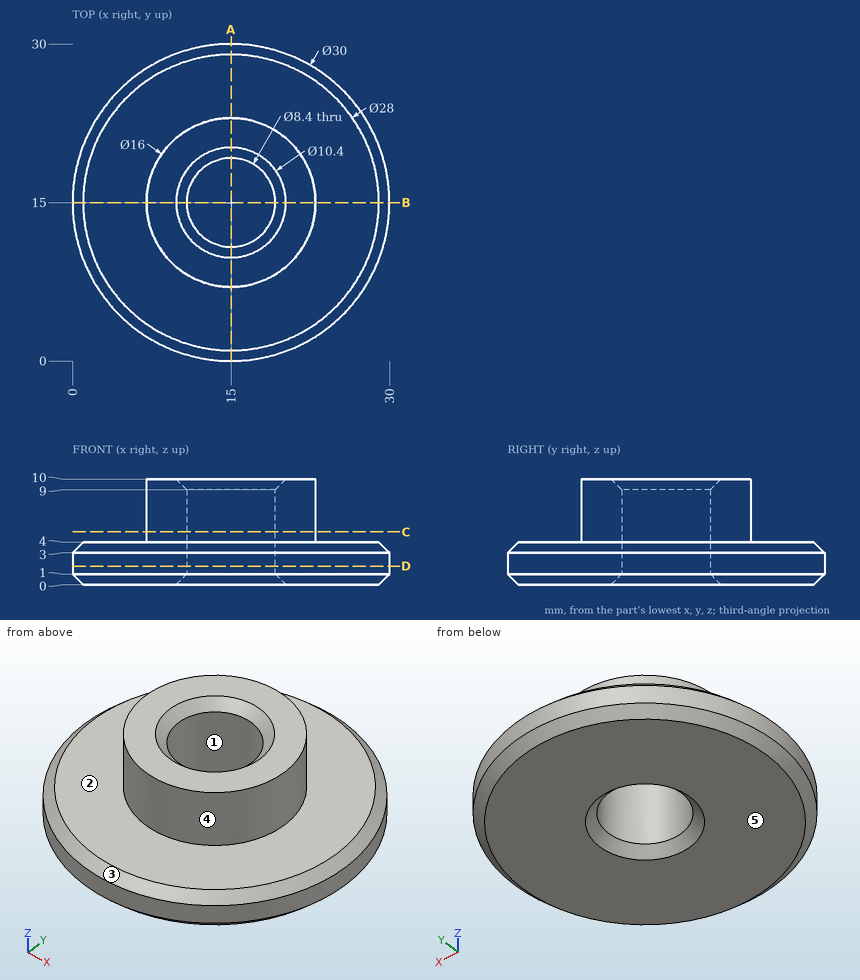
Study the drawing (mm; zero at the part's minimum x, y, z) and answer. A direction names the side the tool comes from. Give positions to 0.01 mm unless a question says otherwise; leave off trailing zeros. Loops run counter-clockwise (first coordinate to the right, second up) from the corner with the lowest first, then second, coordinate; pieces in that order, holes last. Notation, with made-up numbers: (80.5, 49.25) - (86.5, 49.25) arc R18 cw to (86.5, 53.25) - close; hole circle Ø8 at (33.25, 0.5). An arc over 180 degrees is marked (long way). Answer in a Markdown table with one row per item. Add a question column.
Q1. The part is cut by section C-C (z = 5). Determine the outline of the cut face in (x, y).
Q2. The part is cut by section D-D (z = 1.75). Determine the outline of the cut face in (x, y), and give its area (3 significant figures).
Q3. Determine the mould class of the marked faces 1, 2 and 3 for opening direction X: released by +X, released by -X, zero draft, split by the parting line, or undercut.
Q4. The part is cut by section A-A (x = 15). Determine the outline of the cut face in (y, z).
Q5. Consider line 1 along Y through (x, z) = (15, 4.75); line 2 along Z through (x, y) = (19.25, 23); line 3 along Y through (x, z) = (16.5, 5.5). Determine where each line is inside the solid, lowest interval first.
Q6. Each of these flat-tipped pins is pushed along its axis until it touches: P1, Ø6, axis at x = 3.5, y = 15.5, coming from the +Z side; P2, Ø6, axis at x = 18.5, z = 3, coming from the +Y side; P3, Ø1.5, axis at x = 12, z = 2.5, coming from the +Y side. Where does it stop, or does it pass through?
Q7. A tool of negligible diameter and unlimited length cuts with its end or side. For the marked faces 4 and 5, from which of +Z, -Z, +X, -X, +Y, -Y can it reach the whole face along a straight path? Write none if from no direction.
Solution:
| question | item | result |
|---|---|---|
| 1 | outline | circle Ø16 at (15, 15); hole circle Ø8.4 at (15, 15) |
| 2 | outline | circle Ø30 at (15, 15); hole circle Ø8.4 at (15, 15) |
| 2 | area | 651 mm² |
| 3 | face 1 | undercut |
| 3 | face 2 | zero draft |
| 3 | face 3 | split by the parting line |
| 4 | outline | (0, 1) - (1, 0) - (9.8, 0) - (10.8, 1) - (10.8, 9) - (9.8, 10) - (7, 10) - (7, 4) - (1, 4) - (0, 3) - close; (19.2, 1) - (20.2, 0) - (29, 0) - (30, 1) - (30, 3) - (29, 4) - (23, 4) - (23, 10) - (20.2, 10) - (19.2, 9) - close |
| 5 | line 1 | y = 7 to 10.8, 19.2 to 23 |
| 5 | line 2 | z = 0 to 4 |
| 5 | line 3 | y = 7.14 to 11.08, 18.92 to 22.86 |
| 6 | P1 | stops at z = 4 |
| 6 | P2 | stops at y = 29.99 |
| 6 | P3 | stops at y = 29.83 |
| 7 | face 4 | +Z |
| 7 | face 5 | -Z, +X, -X, +Y, -Y |
